```python
from build123d import *

# Parameters (mm, degrees)
F0_W     = 45.339
F0_H     = 38.4048
F1_DEPTH = 3.429
F2_W     = 12.309304
F2_H     = 1.4732
F2_W_2   = 5.751361
F2_H_2   = 10.011873
F3_DEPTH = 25.4
F4_W     = 45.339
F4_H     = 3.429
F5_DEPTH = 25.4


with BuildPart() as f1:
    # F0 (on Top) → F1 (new body)
    with BuildSketch(Plane.XY):
        with Locations((-0.877853, 11.814515)):
            Rectangle(F0_W, F0_H)
    extrude(amount=F1_DEPTH)

    # F2 (on face) → F3 (cut)
    with BuildSketch(Plane.XY.offset(3.429)):
        with Locations((-14.737868, 23.142915)):
            Rectangle(F2_W, F2_H)
        with Locations((12.982161, 23.142915)):
            Rectangle(F2_W, F2_H)
        with Locations((-14.737868, 0.486115)):
            Rectangle(F2_W, F2_H)
        with Locations((12.982161, 0.486115)):
            Rectangle(F2_W, F2_H)
        with Locations((21.791646, 11.814514)):
            Rectangle(F2_W_2, F2_H_2)
    extrude(amount=-F3_DEPTH, mode=Mode.SUBTRACT)

    # F4 (on face) → F5 (join)
    with BuildSketch(Plane(origin=(0, 31.016915, 0), x_dir=(-1, 0, 0), z_dir=(0, 1, 0))):
        with Locations((0.877853, 1.7145)):
            Rectangle(F4_W, F4_H)
    extrude(amount=F5_DEPTH)


solid = f1.part
```
Part model, mm, in its own coordinate system. A direction names the side the tool comes from. Round coordinates to 2 decimals unless told otherwise and drop trailing zeros. Order: outer loops, then holes, each group sorted by start corner. A loop starts at its lowest first (then second) coordinate and runs counter-clockwise, first axis right, second up. Notation, with made-up numbers: M 69.5,53.5 L 81.5,53.5 A11 cw 81.5,58.5 Z; hole C 19,14.5 d2. An arc over 180 degrees is marked long. Put each result on its own line as item: value. Start each with the question number.
1. Drill centre lines: probe 1 along Y at (x, z) = (-18, 2.9); probe 2 along X at (y, z) = (13, 1.4). Where is each one in solid material? Low to high. Write a range as [from, to].
2. Two-plate mould, pull along X, no slides. Class faces 4 (the face through (-23.547, 24, 2)), 5 (the face through (13, 22.406, 2)), 6 (the face through (-15, 23.88, 2)), 7 (the face through (18.916, 12, 2)): +X half, -X half, draft (parallel to the pull), parting line (faces both ways), or undercut.
3. Tool access for faces 1 (the face through (-1, -7.388, 2)), 2 (the face through (19.137, 0, 2)), 3 (the face through (20, 16.82, 2)): list every direction of +Z, -Z, +X, -X, +Y, -Y with a clear straight run to the whole face (end or side of a thin tool).
4. Slice it at B-B on z = 2.75. List the corners of the cut face in (x, y).
5. Drop a flat-ended pin along its axis: pin 1 (1.7 mm diameter, centred on y = 12.5, z = 1, fed in from +X). Give the stop position or say it passes through.
6. Slice it at A-A on x = 16. List the corners of the cut face in (y, z), then the cut area to 3 significant figures.
Findings:
1. probe 1: [-7.39, -0.25], [1.22, 22.41], [23.88, 56.42]
1. probe 2: [-23.55, 18.92]
2. face 4: -X half
2. face 5: undercut
2. face 6: undercut
2. face 7: +X half
3. face 1: +Z, -Z, +X, -X, -Y
3. face 2: +Z, -Z
3. face 3: +Z, -Z, +X
4. outline: M -23.55,-7.39 L 21.79,-7.39 L 21.79,6.81 L 18.92,6.81 L 18.92,16.82 L 21.79,16.82 L 21.79,56.42 L -23.55,56.42 Z; hole M -20.89,-0.25 L -8.58,-0.25 L -8.58,1.22 L -20.89,1.22 Z; hole M -20.89,22.41 L -8.58,22.41 L -8.58,23.88 L -20.89,23.88 Z; hole M 6.83,-0.25 L 19.14,-0.25 L 19.14,1.22 L 6.83,1.22 Z; hole M 6.83,22.41 L 19.14,22.41 L 19.14,23.88 L 6.83,23.88 Z
5. pin 1: x = 18.92
6. outline: M -7.39,0 L -0.25,0 L -0.25,3.43 L -7.39,3.43 Z; M 1.22,0 L 22.41,0 L 22.41,3.43 L 1.22,3.43 Z; M 23.88,0 L 56.42,0 L 56.42,3.43 L 23.88,3.43 Z
6. area: 209 mm2
